Build history of the part. All positions in model axes, mm. Coordinates: 2 decimals unless noted, no trailing zeros. Write each loop counter-clockwise with the first axis right and the second up, starting at its lowest first coordinate (ties: lowest second). Pieces come first, ordered by that corner, then holes. Notation, with made-up numbers: M 88,53.25 L 97,53.25 A24 ccw 97,87.25 Z; hole C -18,5.25 d4. An arc over 180 degrees is marked long. Use CSV: the item, a comma, the result in double quotes. Start each with the question number.
```python
from build123d import *

# Parameters (mm, degrees)
BOSS_EXTRUDE1_DEPTH            = 3.175
M4_CLEARANCE_HOLE1_D           = 4.5
M4_CLEARANCE_HOLE1_CSINK_D     = 4.55
M4_CLEARANCE_HOLE1_CSINK_ANGLE = 90
M8_CLEARANCE_HOLE1_AT_2_COUNT  = 2
M8_CLEARANCE_HOLE1_AT_2_PITCH  = 84
SKETCH9_R                      = 21.275
CENTER_HOLE_DEPTH              = 4.175


with BuildPart() as part:
    # Sketch1 → Boss-Extrude1 (new body)
    with BuildSketch(Plane.XY):
        Polygon((-76.2, 48.26), (-76.2, 44.45), (-76.2, -44.45), (76.2, -44.45), (76.2, 44.45), (76.2, 50.8), align=None)
    extrude(amount=BOSS_EXTRUDE1_DEPTH)

    # M4 Clearance Hole1 (through all)
    with Locations(Plane.XY.offset(3.175)):
        with Locations((0, 38.1), (-66.04, 34.29), (-66.04, -34.29), (0, -38.1), (66.04, -34.29), (66.04, 34.29)):
            CounterSinkHole(M4_CLEARANCE_HOLE1_D / 2, M4_CLEARANCE_HOLE1_CSINK_D / 2, counter_sink_angle=M4_CLEARANCE_HOLE1_CSINK_ANGLE)

    # Sketch11 → M8 Clearance Hole1 (revolve, cut)
    with BuildSketch(Plane(origin=(-42, 0, 3.175), x_dir=(0, -1, 0), z_dir=(1, 0, 0))):
        Polygon((0, 0), (0, 3.175), (4.5, 3.175), (4.5, 0.025), (4.525, 0), align=None)
    m8_clearance_hole1 = revolve(axis=Axis((-42, 0, 9.525), (0, 0, -1)), mode=Mode.SUBTRACT)

    # M8 Clearance Hole1 at 2: M8 Clearance Hole1 ×2
    with Locations(*[(i * M8_CLEARANCE_HOLE1_AT_2_PITCH, 0, 0) for i in range(1, M8_CLEARANCE_HOLE1_AT_2_COUNT)]):
        add(m8_clearance_hole1, mode=Mode.SUBTRACT)

    # Sketch9 → Center Hole (cut, through all)
    with BuildSketch(Plane.XY.offset(3.175)):
        Circle(SKETCH9_R)
    extrude(amount=-CENTER_HOLE_DEPTH, mode=Mode.SUBTRACT)


solid = part.part
```
1. Slice it at D-D (y = 38.1). List the corners of the cut face in (x, z) (3 decimals).
2. Slice it at A-A (x = -42). List the corners of the cut face in (y, z) (3 decimals), and give its area (3 significant figures).
3. Slice it at B-B (y = 0). List the corners of the cut face in (x, z) (3 decimals).
4. Flat gauge pins, fed straight in: pin 1 (6 mm diameter, centred on x = 55.5, y = 35.5, fed in from -Z); pin 2 (2.5 mm diameter, centred on x = -66.04, y = -34.29, fed in from +Z). Where does each tip first touch, or does it go through?
5. Slice it at C-C (x = 0). List the corners of the cut face in (y, z) (3 decimals), and give its area (3 significant figures).
6. Drill centre lines: line 1 along X through (y, z) = (-34.29, 2); line 2 along Y through (x, z) = (0, 2.05) (3 decimals); line 3 along Y through (x, z) = (-67.5, 1.3) (3 decimals). Where is each one in solid material? Low to high. Write a range as from..to.
Established:
1,outline,"M -76.2,0 L -2.25,0 L -2.25,3.15 L -2.275,3.175 L -76.2,3.175 Z; M 2.25,0 L 76.2,0 L 76.2,3.175 L 2.275,3.175 L 2.25,3.15 Z"
2,outline,"M -44.45,0 L -4.5,0 L -4.5,3.15 L -4.525,3.175 L -44.45,3.175 Z; M 4.5,0 L 48.83,0 L 48.83,3.175 L 4.525,3.175 L 4.5,3.15 Z"
2,area,"268 mm2"
3,outline,"M -76.2,0 L -46.5,0 L -46.5,3.15 L -46.525,3.175 L -76.2,3.175 Z; M -37.5,0 L -21.275,0 L -21.275,3.175 L -37.475,3.175 L -37.5,3.15 Z; M 21.275,0 L 37.5,0 L 37.5,3.15 L 37.475,3.175 L 21.275,3.175 Z; M 46.5,0 L 76.2,0 L 76.2,3.175 L 46.525,3.175 L 46.5,3.15 Z"
4,pin 1,"stops at z = 0"
4,pin 2,"passes through"
5,outline,"M -44.45,0 L -40.35,0 L -40.35,3.15 L -40.375,3.175 L -44.45,3.175 Z; M -35.85,0 L -21.275,0 L -21.275,3.175 L -35.825,3.175 L -35.85,3.15 Z; M 21.275,0 L 35.85,0 L 35.85,3.15 L 35.825,3.175 L 21.275,3.175 Z; M 40.35,0 L 49.53,0 L 49.53,3.175 L 40.375,3.175 L 40.35,3.15 Z"
5,area,"135 mm2"
6,line 1,"x = -76.2..-68.29, -63.79..63.79, 68.29..76.2"
6,line 2,"y = -44.45..-40.35, -35.85..-21.275, 21.275..35.85, 40.35..49.53"
6,line 3,"y = -44.45..-36.002, -32.578..32.578, 36.002..48.405"
